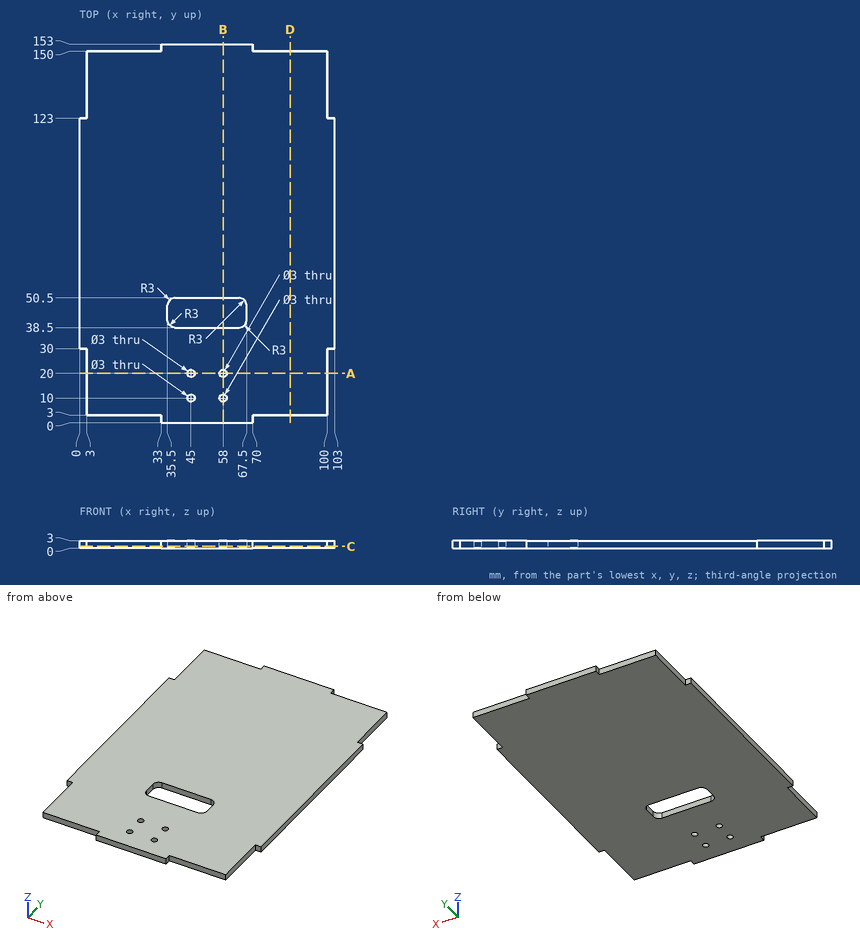
For this review, use the dimensioned drawing (mm, ordinates from the lowest corner) and the shaded views. Give positions to 0.01 mm unless a question says otherwise; leave off trailing zeros. Loops run counter-clockwise (first coordinate to the right, second up) from the corner with the lowest first, then second, coordinate; pieces in that order, holes last. Notation, with made-up numbers: (88.5, 46) -> (99.5, 46) arc R19 cw to (99.5, 63) -> close; hole circle Ø7 at (-34, 74). An arc over 180 degrees is marked (long way). One line per question, with ' | ' between items. Start each with the question number.
(1) We need section B-B (x = 58). State the section outline as (y, z) points.
(2) For line 1 (Y direction, x = 45, z = 1.45); line 2 (X direction, y = 10, z = 1.15); line 3 (Y direction, x = 50, z = 1.65), list the stretches that pass through material, from the lowest coordinate up.
(3) We need section D-D (x = 85). State the section outline as (y, z) points, and give its area (3 significant figures).
(4) We need section A-A (y = 20). State the section outline as (x, z) points.
(5) Insertion check: P1, Ø1.5, axis at y = 2, z = 1.5, coming from the +X side; P2, Ø0.9, axis at y = 135, z = 2, coming from the -X side; P3, Ø0.9, axis at y = 151, z = 2, coming from the -X side. Each pin has a flat end and moves straight along its axis. Give the tip position at first contact, or say it passes through.
(6) We need section C-C (z = 0.75). State how many separate pieces and enclosed holes the cut face has, and give its area (3 significant figures).
The answers:
1) outline: (0, 0) -> (8.5, 0) -> (8.5, 3) -> (0, 3) -> close; (11.5, 0) -> (18.5, 0) -> (18.5, 3) -> (11.5, 3) -> close; (21.5, 0) -> (38.5, 0) -> (38.5, 3) -> (21.5, 3) -> close; (50.5, 0) -> (153, 0) -> (153, 3) -> (50.5, 3) -> close
2) line 1: y = 0 to 8.5, 11.5 to 18.5, 21.5 to 38.5, 50.5 to 153 | line 2: x = 3 to 43.5, 46.5 to 56.5, 59.5 to 100 | line 3: y = 0 to 38.5, 50.5 to 153
3) outline: (3, 0) -> (150, 0) -> (150, 3) -> (3, 3) -> close | area: 441 mm^2
4) outline: (3, 0) -> (43.5, 0) -> (43.5, 3) -> (3, 3) -> close; (46.5, 0) -> (56.5, 0) -> (56.5, 3) -> (46.5, 3) -> close; (59.5, 0) -> (100, 0) -> (100, 3) -> (59.5, 3) -> close
5) P1: stops at x = 70 | P2: stops at x = 3 | P3: stops at x = 33
6) separate pieces: 1 | enclosed holes: 5 | area: 14,600 mm^2
